Build history of the part. All positions in model axes, mm. Round coordinates to 2 decimals unless told otherwise and drop trailing zeros. Loops run counter-clockwise (first coordinate to the right, second up) from the corner with the lowest first, then second, coordinate; pieces in that order, holes last. Notation, with made-up numbers: (58, 38) - (81, 38) arc R30 ccw to (81, 73) - close; hole circle Ø9 at (-35.75, 33). An arc over 180 degrees is marked (long way). Use a Markdown table: item, result.
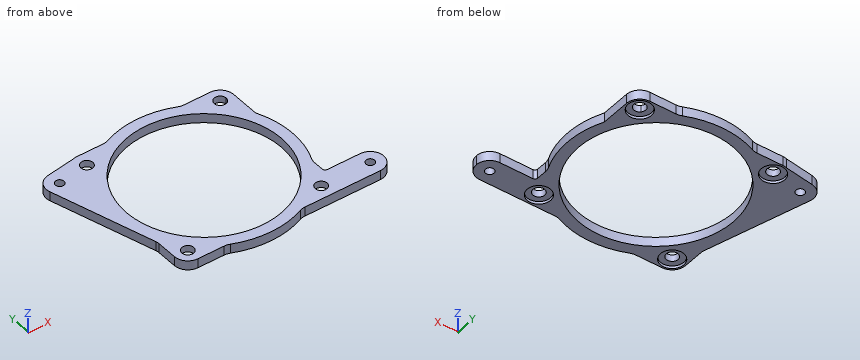
from build123d import *

# Parameters (mm, degrees)
F0_R     = 2.22
F0_R_2   = 29
F0_R_3   = 1.6
F2_DEPTH = 3.5
F3_R     = 4.375
F3_R_2   = 2.22
F4_DEPTH = 1


with BuildPart() as f2:
    # F0 (on Top) → F2 (new body)
    with BuildSketch(Plane.XY):
        with BuildLine():
            Line((-28.0399272842, 48.7993610323), (-26.564868493, 49.0218929201))
            ThreePointArc((-26.564868493, 49.0218929201), (-27.3107436298, 48.965946953), (-28.0399272842, 48.7993610323))
        make_face()
        with BuildLine():
            Line((-16.69420754, 49.0218929201), (-26.564868493, 49.0218929201))
            Line((-26.564868493, 49.0218929201), (-28.0399272842, 48.7993610323))
            Line((-28.0399272842, 48.7993610323), (-38.8670578152, 47.165946953))
            ThreePointArc((-38.8670578152, 47.165946953), (-42.3386518344, 44.9075872285), (-42.9166986895, 40.8066098434))
            Line((-42.9166986895, 40.8066098434), (-31.7693524819, 3.0351716781))
            ThreePointArc((-31.7693524819, 3.0351716781), (-31.6162535325, 2.3348780924), (-31.564868493, 1.6198886013))
            Line((-31.564868493, 1.6198886013), (-31.564868493, -5.9781070799))
            ThreePointArc((-31.564868493, -5.9781070799), (-30.1004023989, -9.5136409858), (-26.564868493, -10.9781070799))
            Line((-26.564868493, -10.9781070799), (-16.69420754, -10.9781070799))
            ThreePointArc((-16.69420754, -10.9781070799), (-15.6812440963, -11.0817916221), (-14.7102921129, -11.3885450552))
            ThreePointArc((-14.7102921129, -11.3885450552), (-1.564868493, -14.1081070799), (11.5805551269, -11.3885450552))
            ThreePointArc((11.5805551269, -11.3885450552), (12.5515071103, -11.0817916221), (13.564470554, -10.9781070799))
            Line((13.564470554, -10.9781070799), (23.435131507, -10.9781070799))
            Line((23.435131507, -10.9781070799), (41.8588173216, -10.9781070799))
            ThreePointArc((41.8588173216, -10.9781070799), (39.4580409401, -10.3640246311), (37.6469744143, -8.6726161862))
            ThreePointArc((37.6469744143, -8.6726161862), (37.5867252108, -8.5760349073), (37.5286903027, -8.4781070799))
            ThreePointArc((37.5286903027, -8.4781070799), (37.5286903027, -3.4781070799), (41.8588173216, -0.9781070799))
            Line((41.8588173216, -0.9781070799), (29.435131507, -0.9781070799))
            ThreePointArc((29.435131507, -0.9781070799), (28.7280247258, -0.6852138611), (28.435131507, 0.0218929201))
            Line((28.435131507, 0.0218929201), (28.435131507, 3.8925538731))
            ThreePointArc((28.435131507, 3.8925538731), (28.5388160493, 4.9055173169), (28.8455694823, 5.8764693002))
            ThreePointArc((28.8455694823, 5.8764693002), (31.5613609993, 19.521712514), (28.435131507, 33.0788093672))
            Line((28.435131507, 33.0788093672), (28.435131507, 44.0218929201))
            ThreePointArc((28.435131507, 44.0218929201), (26.9706654129, 47.5574268261), (23.435131507, 49.0218929201))
            Line((23.435131507, 49.0218929201), (13.564470554, 49.0218929201))
            ThreePointArc((13.564470554, 49.0218929201), (12.5515071103, 49.1255774624), (11.5805551269, 49.4323308955))
            ThreePointArc((11.5805551269, 49.4323308955), (-1.564868493, 52.1518929201), (-14.7102921129, 49.4323308955))
            ThreePointArc((-14.7102921129, 49.4323308955), (-15.6812440963, 49.1255774624), (-16.69420754, 49.0218929201))
        make_face()
        with Locations((-26.5610932079, -5.9743317948)):
            Circle(F0_R, mode=Mode.SUBTRACT)
        with Locations((23.4313562219, -5.9743317948)):
            Circle(F0_R, mode=Mode.SUBTRACT)
        with Locations((-1.564868493, 19.0218929201)):
            Circle(F0_R_2, mode=Mode.SUBTRACT)
        with Locations((-38.1211826784, 42.2218929201)):
            Circle(F0_R_3, mode=Mode.SUBTRACT)
        with Locations((-26.561093208, 44.0181176351)):
            Circle(F0_R, mode=Mode.SUBTRACT)
        with BuildLine():
            ThreePointArc((25.6513562219, 44.0181176351), (24.2809134408, 41.9671050725), (21.8615791662, 42.4483405824))
            ThreePointArc((21.8615791662, 42.4483405824), (22.5817990031, 46.0691301977), (25.6513562219, 44.0181176351))
        make_face(mode=Mode.SUBTRACT)
        with BuildLine():
            ThreePointArc((46.8588173216, -5.9781070799), (45.3943512276, -2.4425731739), (41.8588173216, -0.9781070799))
            ThreePointArc((41.8588173216, -0.9781070799), (37.5286903027, -3.4781070799), (37.5286903027, -8.4781070799))
            ThreePointArc((37.5286903027, -8.4781070799), (37.5867252108, -8.5760349073), (37.6469744143, -8.6726161862))
            ThreePointArc((37.6469744143, -8.6726161862), (39.4580409401, -10.3640246311), (41.8588173216, -10.9781070799))
            ThreePointArc((41.8588173216, -10.9781070799), (45.3943512276, -9.5136409858), (46.8588173216, -5.9781070799))
        make_face()
        with Locations((41.8588173216, -5.9781070799)):
            Circle(F0_R_3, mode=Mode.SUBTRACT)
    extrude(amount=F2_DEPTH)

    # F3 (on face) → F4 (cut)
    with BuildSketch(Plane(origin=(0, 0, 0), x_dir=(1, 0, 0), z_dir=(0, 0, -1))):
        with Locations((23.4313562219, 5.9743317948)):
            Circle(F3_R)
        with Locations((23.4313562219, 5.9743317948)):
            Circle(F3_R_2, mode=Mode.SUBTRACT)
        with Locations((-26.5610932079, 5.9743317948)):
            Circle(F3_R)
        with Locations((-26.5610932079, 5.9743317948)):
            Circle(F3_R_2, mode=Mode.SUBTRACT)
        with Locations((-26.561093208, -44.0181176351)):
            Circle(F3_R)
        with Locations((-26.561093208, -44.0181176351)):
            Circle(F3_R_2, mode=Mode.SUBTRACT)
        with Locations((23.4313562219, -44.0181176351)):
            Circle(F3_R)
        with Locations((23.4313562219, -44.0181176351)):
            Circle(F3_R_2, mode=Mode.SUBTRACT)
        with Locations((-26.5610932079, 5.9743317948)):
            Circle(F3_R_2)
        with Locations((23.4313562219, 5.9743317948)):
            Circle(F3_R_2)
        with Locations((23.4313562219, -44.0181176351)):
            Circle(F3_R_2)
        with Locations((-26.561093208, -44.0181176351)):
            Circle(F3_R_2)
    extrude(amount=-F4_DEPTH, mode=Mode.SUBTRACT)


solid = f2.part
Q1. Cut at C-C, the plane z = 2.85. Count the separate pieces of the cut face and the enclosed holes in it, plus the area to 3 significant figures.
Results found:
| item | result |
|---|---|
| separate pieces | 1 |
| enclosed holes | 7 |
| area | 1,510 mm2 |
Q2. Cut at A-A, the plane y = 29. List the corners of the cut face in (x, z).
Results found:
| item | result |
|---|---|
| outline | (-39.43, 0) - (-28.79, 0) - (-28.79, 3.5) - (-39.43, 3.5) - close; (25.66, 0) - (30.03, 0) - (30.03, 3.5) - (25.66, 3.5) - close |
Q3. Cut at B-B, the plane x = -9.5. List the corners of the cut face in (y, z).
Results found:
| item | result |
|---|---|
| outline | (-13.14, 0) - (-8.87, 0) - (-8.87, 3.5) - (-13.14, 3.5) - close; (46.92, 0) - (51.19, 0) - (51.19, 3.5) - (46.92, 3.5) - close |
Q4. Cut at D-D, the plane x = -35.5. List the corners of the cut face in (y, z), plus the area to 3 significant figures.
Results found:
| item | result |
|---|---|
| outline | (15.68, 0) - (47.67, 0) - (47.67, 3.5) - (15.68, 3.5) - close |
| area | 112 mm2 |
Q5. Probe line 1 (X direction, y = -3, z = 0.9); line 2 (X direction, y = -2, z = 0.45); line 3 (X direction, y = -7, z = 1.2). List the from-to ranges inside material, lowest first.
Results found:
| item | result |
|---|---|
| line 1 | x = -31.56 to -29.77, -23.35 to -20.43, 17.3 to 20.22, 26.64 to 45.88 |
| line 2 | x = -31.56 to -28.39, -24.73 to -21.54, 18.41 to 21.6, 25.26 to 44.89 |
| line 3 | x = -31.46 to -28.53, -24.59 to -14.37, 11.24 to 21.46, 25.4 to 40.63, 43.09 to 46.75 |
Q6. Drop flat-ended pins along their axis: pin 1 (7 mm diameter, centred on x = 23, y = 44.5, fed in from -Z); pin 2 (1.8 mm diameter, centred on x = -23.5, z = 2, fed in from -Y); pin 3 (10 mm diameter, centred on x = -26.56, y = -5.97, fed in from +Z); pin 4 (2 mm diameter, centred on y = 0, z = 2.5, fed in from -X). Give the stop position or say it passes through.
Results found:
| item | result |
|---|---|
| pin 1 | stops at z = 1 |
| pin 2 | stops at y = -10.98 |
| pin 3 | stops at z = 3.5 |
| pin 4 | stops at x = -31.56 |
